from build123d import *

# Parameters (mm, degrees)
SKETCH1_W           = 164.87
SKETCH1_H           = 104.3
SKETCH1_W_2         = 154.97
SKETCH1_H_2         = 94.47
BOSS_EXTRUDE1_DEPTH = 12
CUT_EXTRUDE3_REACH  = 229.35
SKETCH2_R           = 1.25
BOSS_EXTRUDE2_START = -13.2
BOSS_EXTRUDE2_DEPTH = 1.2
CUT_EXTRUDE4_REACH  = 229.416
SKETCH13_W          = 166.97
SKETCH13_H          = 131.47
CUT_EXTRUDE5_START  = -2
CUT_EXTRUDE5_DEPTH  = 2


with BuildPart() as part:
    # Sketch1 → Boss-Extrude1 (new body)
    # profile 1 of 3: a face of its own
    with BuildSketch(Plane(origin=(0, 0, 0), x_dir=(1, 0, 0), z_dir=(0, 1, 0))):
        with BuildLine():
            ThreePointArc((174.2, 7.54), (176.321320344, 6.661320344), (177.2, 4.54))
            Line((177.2, 4.54), (177.2, -138.93))
            ThreePointArc((177.2, -138.93), (176.321320344, -141.051320344), (174.2, -141.93))
            Line((174.2, -141.93), (-4.77, -141.93))
            ThreePointArc((-4.77, -141.93), (-6.891320344, -141.051320344), (-7.77, -138.93))
            Line((-7.77, -138.93), (-7.77, 4.54))
            ThreePointArc((-7.77, 4.54), (-6.891320344, 6.661320344), (-4.77, 7.54))
            Line((-4.77, 7.54), (174.2, 7.54))
        make_face()
        with Locations((82.435, -52.15)):
            Rectangle(SKETCH1_W, SKETCH1_H, mode=Mode.SUBTRACT)
    # profile 2 of 3: a face of its own
    with BuildSketch(Plane(origin=(0, 0, 0), x_dir=(1, 0, 0), z_dir=(0, 1, 0))):
        with Locations((82.435, -52.15)):
            Rectangle(SKETCH1_W, SKETCH1_H)
        with Locations((84.715, -54.695)):
            Rectangle(SKETCH1_W_2, SKETCH1_H_2, mode=Mode.SUBTRACT)
    # profile 3 of 3: a face of its own
    with BuildSketch(Plane(origin=(0, 0, 0), x_dir=(1, 0, 0), z_dir=(0, 1, 0))):
        with Locations((84.715, -54.695)):
            Rectangle(SKETCH1_W_2, SKETCH1_H_2)
    extrude(amount=-BOSS_EXTRUDE1_DEPTH)

    # Sketch2 → Cut-Extrude3 (cut, up to next)
    with BuildSketch(Plane.XZ.offset(12), mode=Mode.PRIVATE) as cut_extrude3_sk1:
        with Locations(Location((172.7, -3.04, 0), (0, 0, 270))):
            Circle(SKETCH2_R)
    cut_extrude3_tool1 = extrude(cut_extrude3_sk1.sketch, amount=-CUT_EXTRUDE3_REACH, mode=Mode.PRIVATE) & part.part
    # Sketch2 → Cut-Extrude3 (cut, up to next)
    with BuildSketch(Plane.XZ.offset(12), mode=Mode.PRIVATE) as cut_extrude3_sk2:
        with Locations(Location((114.05, -3.04, 0), (0, 0, 270))):
            Circle(SKETCH2_R)
    cut_extrude3_tool2 = extrude(cut_extrude3_sk2.sketch, amount=-CUT_EXTRUDE3_REACH, mode=Mode.PRIVATE) & part.part
    # Sketch2 → Cut-Extrude3 (cut, up to next)
    with BuildSketch(Plane.XZ.offset(12), mode=Mode.PRIVATE) as cut_extrude3_sk3:
        with Locations(Location((-3.27, -3.04, 0), (0, 0, 270))):
            Circle(SKETCH2_R)
    cut_extrude3_tool3 = extrude(cut_extrude3_sk3.sketch, amount=-CUT_EXTRUDE3_REACH, mode=Mode.PRIVATE) & part.part
    # Sketch2 → Cut-Extrude3 (cut, up to next)
    with BuildSketch(Plane.XZ.offset(12), mode=Mode.PRIVATE) as cut_extrude3_sk4:
        with Locations(Location((-3.27, 83.94, 0), (0, 0, 270))):
            Circle(SKETCH2_R)
    cut_extrude3_tool4 = extrude(cut_extrude3_sk4.sketch, amount=-CUT_EXTRUDE3_REACH, mode=Mode.PRIVATE) & part.part
    # Sketch2 → Cut-Extrude3 (cut, up to next)
    with BuildSketch(Plane.XZ.offset(12), mode=Mode.PRIVATE) as cut_extrude3_sk5:
        with Locations(Location((-3.27, 137.43, 0), (0, 0, 270))):
            Circle(SKETCH2_R)
    cut_extrude3_tool5 = extrude(cut_extrude3_sk5.sketch, amount=-CUT_EXTRUDE3_REACH, mode=Mode.PRIVATE) & part.part
    # Sketch2 → Cut-Extrude3 (cut, up to next)
    with BuildSketch(Plane.XZ.offset(12), mode=Mode.PRIVATE) as cut_extrude3_sk6:
        with Locations(Location((55.38, 137.43, 0), (0, 0, 270))):
            Circle(SKETCH2_R)
    cut_extrude3_tool6 = extrude(cut_extrude3_sk6.sketch, amount=-CUT_EXTRUDE3_REACH, mode=Mode.PRIVATE) & part.part
    # Sketch2 → Cut-Extrude3 (cut, up to next)
    with BuildSketch(Plane.XZ.offset(12), mode=Mode.PRIVATE) as cut_extrude3_sk7:
        with Locations(Location((114.05, 137.43, 0), (0, 0, 270))):
            Circle(SKETCH2_R)
    cut_extrude3_tool7 = extrude(cut_extrude3_sk7.sketch, amount=-CUT_EXTRUDE3_REACH, mode=Mode.PRIVATE) & part.part
    # Sketch2 → Cut-Extrude3 (cut, up to next)
    with BuildSketch(Plane.XZ.offset(12), mode=Mode.PRIVATE) as cut_extrude3_sk8:
        with Locations(Location((172.7, 137.43, 0), (0, 0, 270))):
            Circle(SKETCH2_R)
    cut_extrude3_tool8 = extrude(cut_extrude3_sk8.sketch, amount=-CUT_EXTRUDE3_REACH, mode=Mode.PRIVATE) & part.part
    # Sketch2 → Cut-Extrude3 (cut, up to next)
    with BuildSketch(Plane.XZ.offset(12), mode=Mode.PRIVATE) as cut_extrude3_sk9:
        with Locations(Location((172.7, 83.94, 0), (0, 0, 270))):
            Circle(SKETCH2_R)
    cut_extrude3_tool9 = extrude(cut_extrude3_sk9.sketch, amount=-CUT_EXTRUDE3_REACH, mode=Mode.PRIVATE) & part.part
    # Sketch2 → Cut-Extrude3 (cut, up to next)
    with BuildSketch(Plane.XZ.offset(12), mode=Mode.PRIVATE) as cut_extrude3_sk10:
        with Locations(Location((172.7, 40.45, 0), (0, 0, 270))):
            Circle(SKETCH2_R)
    cut_extrude3_tool10 = extrude(cut_extrude3_sk10.sketch, amount=-CUT_EXTRUDE3_REACH, mode=Mode.PRIVATE) & part.part
    # Sketch2 → Cut-Extrude3 (cut, up to next)
    with BuildSketch(Plane.XZ.offset(12), mode=Mode.PRIVATE) as cut_extrude3_sk11:
        with Locations(Location((55.38, -3.04, 0), (0, 0, 270))):
            Circle(SKETCH2_R)
    cut_extrude3_tool11 = extrude(cut_extrude3_sk11.sketch, amount=-CUT_EXTRUDE3_REACH, mode=Mode.PRIVATE) & part.part
    # Sketch2 → Cut-Extrude3 (cut, up to next)
    with BuildSketch(Plane.XZ.offset(12), mode=Mode.PRIVATE) as cut_extrude3_sk12:
        with Locations(Location((-3.27, 40.45, 0), (0, 0, 270))):
            Circle(SKETCH2_R)
    cut_extrude3_tool12 = extrude(cut_extrude3_sk12.sketch, amount=-CUT_EXTRUDE3_REACH, mode=Mode.PRIVATE) & part.part
    add(cut_extrude3_tool1.solids().sort_by_distance((172.7, -12, -3.04))[0], mode=Mode.SUBTRACT)
    add(cut_extrude3_tool2.solids().sort_by_distance((114.05, -12, -3.04))[0], mode=Mode.SUBTRACT)
    add(cut_extrude3_tool3.solids().sort_by_distance((-3.27, -12, -3.04))[0], mode=Mode.SUBTRACT)
    add(cut_extrude3_tool4.solids().sort_by_distance((-3.27, -12, 83.94))[0], mode=Mode.SUBTRACT)
    add(cut_extrude3_tool5.solids().sort_by_distance((-3.27, -12, 137.43))[0], mode=Mode.SUBTRACT)
    add(cut_extrude3_tool6.solids().sort_by_distance((55.38, -12, 137.43))[0], mode=Mode.SUBTRACT)
    add(cut_extrude3_tool7.solids().sort_by_distance((114.05, -12, 137.43))[0], mode=Mode.SUBTRACT)
    add(cut_extrude3_tool8.solids().sort_by_distance((172.7, -12, 137.43))[0], mode=Mode.SUBTRACT)
    add(cut_extrude3_tool9.solids().sort_by_distance((172.7, -12, 83.94))[0], mode=Mode.SUBTRACT)
    add(cut_extrude3_tool10.solids().sort_by_distance((172.7, -12, 40.45))[0], mode=Mode.SUBTRACT)
    add(cut_extrude3_tool11.solids().sort_by_distance((55.38, -12, -3.04))[0], mode=Mode.SUBTRACT)
    add(cut_extrude3_tool12.solids().sort_by_distance((-3.27, -12, 40.45))[0], mode=Mode.SUBTRACT)

    # Sketch12 → Boss-Extrude2 (add)
    with BuildSketch(Plane.XZ.offset(12).offset(BOSS_EXTRUDE2_START)):
        with BuildLine():
            Line((-4.77, -7.54), (174.2, -7.54))
            ThreePointArc((174.2, -7.54), (176.321320344, -6.661320344), (177.2, -4.54))
            Line((177.2, -4.54), (177.2, 138.93))
            ThreePointArc((177.2, 138.93), (176.321320344, 141.051320344), (174.2, 141.93))
            Line((174.2, 141.93), (-4.77, 141.93))
            ThreePointArc((-4.77, 141.93), (-6.891320344, 141.051320344), (-7.77, 138.93))
            Line((-7.77, 138.93), (-7.77, -4.54))
            ThreePointArc((-7.77, -4.54), (-6.891320344, -6.661320344), (-4.77, -7.54))
        make_face()
        with BuildLine():
            ThreePointArc((174.2, -6.79), (175.790990258, -6.130990258), (176.45, -4.54))
            Line((176.45, -4.54), (176.45, 138.93))
            ThreePointArc((176.45, 138.93), (175.790990258, 140.520990258), (174.2, 141.18))
            Line((174.2, 141.18), (-4.77, 141.18))
            ThreePointArc((-4.77, 141.18), (-6.360990258, 140.520990258), (-7.02, 138.93))
            Line((-7.02, 138.93), (-7.02, -4.54))
            ThreePointArc((-7.02, -4.54), (-6.360990258, -6.130990258), (-4.77, -6.79))
            Line((-4.77, -6.79), (174.2, -6.79))
        make_face(mode=Mode.SUBTRACT)
    extrude(amount=BOSS_EXTRUDE2_DEPTH)

    # Sketch13 → Cut-Extrude4 (cut, up to next)
    with BuildSketch(Plane.XZ.offset(12), mode=Mode.PRIVATE) as cut_extrude4_sk1:
        with Locations((84.715, 67.195)):
            Rectangle(SKETCH13_W, SKETCH13_H)
    cut_extrude4_tool1 = extrude(cut_extrude4_sk1.sketch, amount=-CUT_EXTRUDE4_REACH, mode=Mode.PRIVATE) & part.part
    add(cut_extrude4_tool1.solids().sort_by_distance((84.715, -12, 67.195))[0], mode=Mode.SUBTRACT)

    # Sketch12<4> → Cut-Extrude5 (cut)
    with BuildSketch(Plane.XZ.offset(12).offset(CUT_EXTRUDE5_START)):
        with BuildLine():
            Line((-4.77, -7.54), (174.2, -7.54))
            ThreePointArc((174.2, -7.54), (176.321320344, -6.661320344), (177.2, -4.54))
            Line((177.2, -4.54), (177.2, 138.93))
            ThreePointArc((177.2, 138.93), (176.321320344, 141.051320344), (174.2, 141.93))
            Line((174.2, 141.93), (-4.77, 141.93))
            ThreePointArc((-4.77, 141.93), (-6.891320344, 141.051320344), (-7.77, 138.93))
            Line((-7.77, 138.93), (-7.77, -4.54))
            ThreePointArc((-7.77, -4.54), (-6.891320344, -6.661320344), (-4.77, -7.54))
        make_face()
        with BuildLine():
            ThreePointArc((174.2, -6.79), (175.790990258, -6.130990258), (176.45, -4.54))
            Line((176.45, -4.54), (176.45, 138.93))
            ThreePointArc((176.45, 138.93), (175.790990258, 140.520990258), (174.2, 141.18))
            Line((174.2, 141.18), (-4.77, 141.18))
            ThreePointArc((-4.77, 141.18), (-6.360990258, 140.520990258), (-7.02, 138.93))
            Line((-7.02, 138.93), (-7.02, -4.54))
            ThreePointArc((-7.02, -4.54), (-6.360990258, -6.130990258), (-4.77, -6.79))
            Line((-4.77, -6.79), (174.2, -6.79))
        make_face(mode=Mode.SUBTRACT)
    extrude(amount=CUT_EXTRUDE5_DEPTH, mode=Mode.SUBTRACT)


solid = part.part
Can you work these out from the model? Positions are in its coordinate system, mm. A direction names the side the tool comes from. Give positions to 0.01 mm unless a question says otherwise; leave off trailing zeros. Order: outer loops, then holes, each group sorted by start corner. A loop starts at its lowest first (then second) coordinate and runs counter-clockwise, first axis right, second up. Notation, with made-up numbers: M 87.25,79 L 107.25,79 A14 ccw 107.25,95 Z; hole C 31.5,-35 d4. An arc over 180 degrees is marked long. Use one line per item in the form item = value.
Item 1: For faces 1 (the flat face through (84, 0, 1)), 2 (the flat face through (84, -6, 132.93)), 3 (the flat face through (177.2, -4, 66)), which set-ups out of +Z, -Z, +X, -X, +Y, -Y let a thin tool reach every point of the face, with its end or its side?
Values follow:
face_1 = +Y
face_2 = +Y, -Y
face_3 = +Z, -Z, +X, +Y, -Y
Item 2: Thinking about a two-plate mould opening in Z: for faces 4 (the flat face through (84, -6, 1.46)), 5 (the flat face through (83, -4, -7.54)), 6 (the flat face through (-7.77, -4, 68)), 7 (the flat face through (168.2, -6, 66)), which applies, pulls with the +Z half, pulls with the -Z half, needs draft (parallel to the pull), parting line crosses it, or undercut?
Values follow:
face_4 = undercut
face_5 = pulls with the -Z half
face_6 = needs draft
face_7 = undercut
Item 3: Will these pins go through, and if not, where does the flat tip stop? pin 1 Ø3 at (x, z) = (-3.27, 40.45) entering from +Y; pin 2 Ø0.6 at (x, y) = (115.5, -11.5) entering from -Z; pin 3 Ø0.6 at (x, y) = (75.5, -11) entering from +Z.
Values follow:
pin_1 = 0
pin_2 = -6.79
pin_3 = 141.18
Item 4: If we section it at C-C, the plane y = -7.75: Count the separate pieces of the cut face and the enclosed holes in it, and give its area (3 significant figures).
Values follow:
separate_pieces = 1
enclosed_holes = 13
area = 5,630 mm^2
Item 5: If we section it at A-A, the plane x = 155.5: Write out the boundary of the cut face in (y, z), and give its area (3 significant figures).
Values follow:
outline = M -12,-6.79 L -10,-6.79 L -10,-7.54 L 1.2,-7.54 L 1.2,-6.79 L 0,-6.79 L 0,1.46 L -12,1.46 Z; M -12,132.93 L 0,132.93 L 0,141.18 L 1.2,141.18 L 1.2,141.93 L -10,141.93 L -10,141.18 L -12,141.18 Z
area = 215 mm^2
Item 6: If I drill on line 1 along X through (y, z) = (-4.25, -3.04); line 2 along X through (y, z) = (-3.5, 83.94); line 3 along Z through (x, y) = (114, -4), over which ranges is the centre line in solid material (lowest first)? Write a range as [from, to].
Values follow:
line_1 = [-7.77, -4.52], [-2.02, 54.13], [56.63, 112.8], [115.3, 171.45], [173.95, 177.2]
line_2 = [-7.77, -4.52], [-2.02, 1.23], [168.2, 171.45], [173.95, 177.2]
line_3 = [-7.54, -4.29], [-1.79, 1.46], [132.93, 136.18], [138.68, 141.93]
Item 7: If we section it at B-B, the plane z = 97: Write out the boundary of the cut face in (x, y), and give its area (3 significant figures).
Values follow:
outline = M -7.77,-10 L -7.02,-10 L -7.02,-12 L 1.23,-12 L 1.23,0 L -7.02,0 L -7.02,1.2 L -7.77,1.2 Z; M 168.2,-12 L 176.45,-12 L 176.45,-10 L 177.2,-10 L 177.2,1.2 L 176.45,1.2 L 176.45,0 L 168.2,0 Z
area = 215 mm^2
